Geometry check sheet. Reference: drawing and pictorial views, mm from the part's lowest x, y, z. Give positions to 0.01 mm unless a question says otherwise; leave off trailing zeros. Write each loop counter-clockwise with the first axis right and the second up, starting at its lowest first coordinate (ties: lowest second). Pieces come first, ordered by that corner, then holes. Notation, with made-up numbers: M -16,-12 L 21,-12 A23 cw 21,3 Z; hole C 17,52 d9. An arc over 180 degrees is marked long. Answer as a JSON object with one key per item and string values.
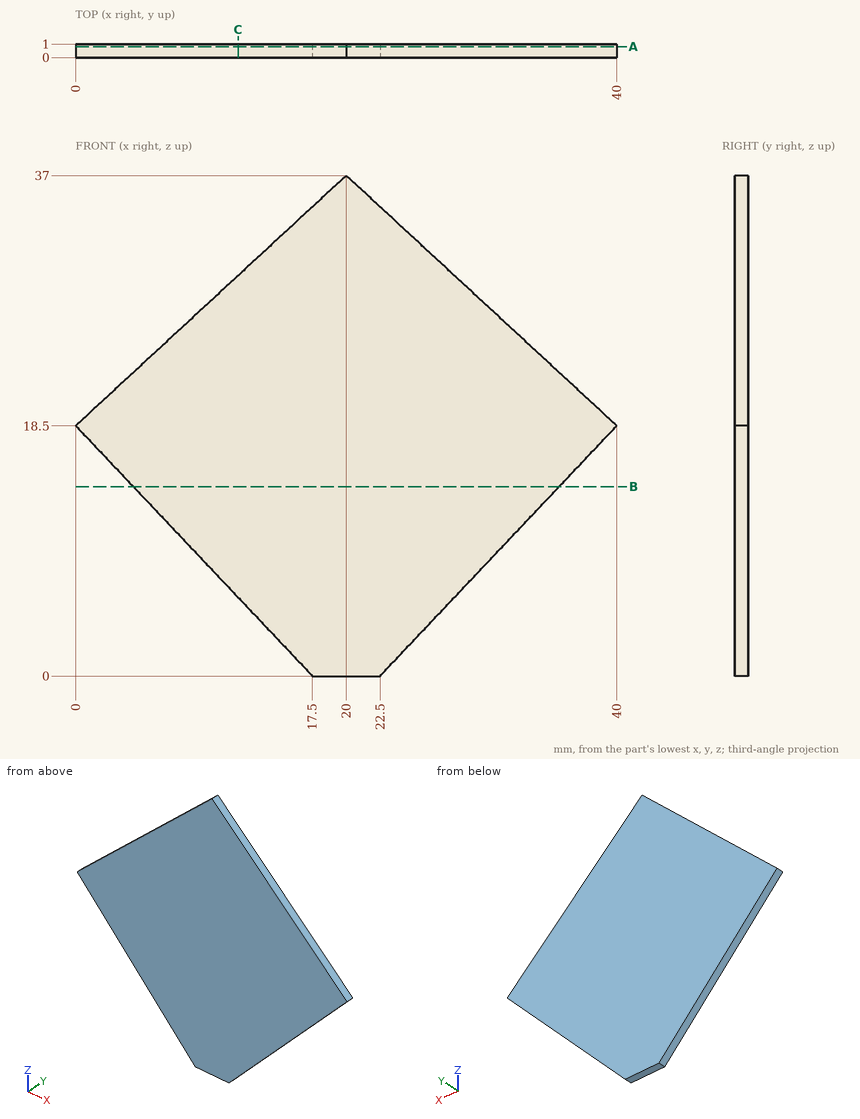
1) Section check B-B on z = 14. Record the boundary of the cut face in (x, y), and give its area (3 significant figures).
Completed:
{"outline": "M 4.26,0 L 35.74,0 L 35.74,1 L 4.26,1 Z", "area": "31.5 mm2"}
2) Section check A-A on y = 0.8. Record the boundary of the cut face in (x, z), and give its area (3 significant figures).
Completed:
{"outline": "M 0,18.5 L 17.5,0 L 22.5,0 L 40,18.5 L 20,37 Z", "area": "786 mm2"}
3) Section check C-C on x = 12. Record the boundary of the cut face in (y, z), and give its area (3 significant figures).
Completed:
{"outline": "M 0,5.81 L 1,5.81 L 1,29.6 L 0,29.6 Z", "area": "23.8 mm2"}
4) Thickness scan on L1, parallel to Z at x = 19, y = 0.95 (3 decimals); L2, parallel to X at y = 0.65, z = 27; L3, parallel to Z at x = 35, y = 0.45 (3 decimals). Record the ranges inside material, lowest first.
Completed:
{"L1": "z = 0 to 36.075", "L2": "x = 9.19 to 30.81", "L3": "z = 13.214 to 23.125"}
